Check sheet for the modelled part. Datum: model origin and axes. Units: mm. Face numbers are marked on the shaded views. A direction names the side the tool comes from. Round coordinates to 2 decimals unless told otherwise and drop trailing zeros. Write each loop counter-clockwise with the first axis right and the second up, starting at its lowest first coordinate (ties: lowest second). Pieces come first, ordered by that corner, then holes. Notation, with made-up numbers: M 73,-21 L 77,-21 A20 ccw 77,11 Z; hole C -37.75,58.5 d9. An arc over 180 degrees is marked long. Put each result on its own line as item: value.
Autodesk Inventor part; units mm, degrees
ref_plane "YZ Plane" through (0, 0, 0) normal (1, 0, 0) x (0, 1, 0)
ref_plane "XZ Plane" through (0, 0, 0) normal (0, 1, 0) x (-1, 0, 0)
ref_plane "XY Plane" through (0, 0, 0) normal (0, 0, 1) x (1, 0, 0)
sketch "Sketch1" plane through (0, 0, 0) normal (0, 1, 0) x (-1, 0, 0)
  line L0 (-15, 20.25) -> (15, 20.25)
  line L1 (15, 20.25) -> (15, -20.25)
  line L2 (15, -20.25) -> (-15, -20.25)
  line L3 (-15, -20.25) -> (-15, 20.25)
  line L4 (-15, 20.25) -> (15, -20.25) construction
  line L5 (15, 20.25) -> (-15, -20.25) construction
  point P0 (0, 0)
  dimension "d0" = 30
  dimension "d1" = 40.5
extrude "Plate1" add sketch "Sketch1" along normal blind 1.5
sketch "Sketch2" plane through (-15, 0, -21.75) normal (0, 0, 1) x (1, 0, 0)
  line L0 (30, 0) -> (0, 0)
  line L1 (0, 0) -> (0, 25)
  line L2 (0, 25) -> (30, 25)
  line L3 (30, 25) -> (30, 0)
edge flange "Flange1" height 25 angle 90 thickness 1.5 bend radius 0.31 thickness toward (0, 0, 1) relief tear relief width 1.5 relief depth 0.75 corner gap 0.31 corner form 0 edges at (0, 1.5, -20.25) (0, 1.5, 20.25) wall of the first edge with corners at (15, 0, -21.75) (-15, 0, -21.75) (-15, 25, -21.75) (15, 25, -21.75)
bend "Bend1"
corner "Corner1"
equation "\"d2\" = Thickness"
equation "\"d3\" = BendReliefWidth"
equation "\"d4\" = BendReliefDepth"
equation "\"d5\" = MinimumRemnant"
equation "\"d6\" = TransitionRadius"
equation "\"d9\" = BendRadius"
equation "\"d10\" = CornerReliefSize"
equation "\"d11\" = GapSize"
equation "\"d12\" = JacobiRadiusSize"
equation "\"BendReliefWidth\" = Thickness"
equation "\"BendReliefDepth\" = 0.5 * Thickness"
equation "\"CornerReliefSize\" = 4 * Thickness"
equation "\"MinimumRemnant\" = 2 * Thickness"
equation "\"TransitionRadius\" = BendRadius"
equation "\"JacobiRadiusSize\" = BendRadius"
equation "\"GapSize\" = Thickness"
properties part number "chanhui" material "Aluminum 6061-AHC"
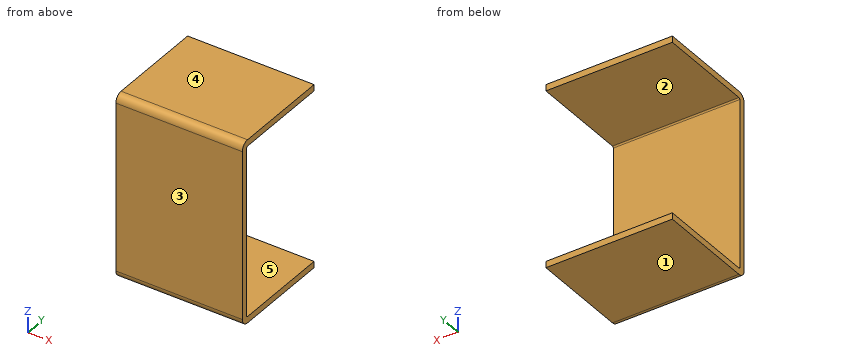
1. Cross-section at A-A (y = 12.5). Enter the section's corners in (x, z).
Computed values:
outline: M -15,-21.75 L 15,-21.75 L 15,-20.25 L -15,-20.25 Z; M -15,20.25 L 15,20.25 L 15,21.75 L -15,21.75 Z
2. Depth check by flat-ended pin: pin 1 Ø2 at (x, z) = (12, 7) entering from -Y. Enter the tip coordinate at first touch or a pass-through.
Computed values:
pin 1: stops at y = 0
3. Scan lines: probe 1 along Z at (x, y) = (-11.5, 3.5); probe 2 along Y at (x, z) = (-5.75, -10). Record each from-to range of solid material in increasing order.
Computed values:
probe 1: z = -21.75 to -20.25, 20.25 to 21.75
probe 2: y = 0 to 1.5
4. Cross-section at C-C (z = -2). Enter the section's corners in (x, y).
Computed values:
outline: M -15,0 L 15,0 L 15,1.5 L -15,1.5 Z
5. Release check for a two-part mould opening along Z. For the marked faces 1, 2 and 3 record: +Z half, -Z half, draft (parallel to the pull), parting line (faces both ways), or undercut.
Computed values:
face 1: -Z half
face 2: undercut
face 3: draft
6. Cross-section at B-B (x = -8.75). Enter the section's corners in (y, z), then the cut area to 3 significant figures.
Computed values:
outline: M 0,-19.94 A1.81 ccw 1.81,-21.75 L 25,-21.75 L 25,-20.25 L 1.81,-20.25 A0.31 cw 1.5,-19.94 L 1.5,19.94 A0.31 cw 1.81,20.25 L 25,20.25 L 25,21.75 L 1.81,21.75 A1.81 ccw 0,19.94 Z
area: 134 mm2
7. Access from +Z, -Z, +X, -X, +Y, -Y to the whole of each face (thin tool, end or side, straight path). Record for the marked faces 4 and 5.
Computed values:
face 4: +Z, +X, -X, +Y, -Y
face 5: +X, -X, +Y
